Model file for the job. Use its own axes, mm. Round coordinates to 2 decimals unless told otherwise and drop trailing zeros. Order: outer loops, then holes, each group sorted by start corner. A loop starts at its lowest first (then second) coordinate and runs counter-clockwise, first axis right, second up. Notation, with made-up numbers: (-24.75, 15.5) - (2.25, 15.5) arc R29 ccw to (2.25, 37.5) - close; hole circle Ø9 at (0, -0.75). An arc over 180 degrees is marked (long way). Use one line per item in the form item = value.
from build123d import *

# Parameters (mm, degrees)
BOSS_EXTRUDE1_DEPTH  = 22
FILLET1_R            = 5
M4_CLEARANCE_HOLE1_D = 4.3
SKETCH5_R            = 11
CUT_EXTRUDE1_DEPTH   = 22


with BuildPart() as part:
    # Sketch1 → Boss-Extrude1 (new body)
    with BuildSketch(Plane.XY):
        Polygon((0, -21.647844006), (15.307337295, -15.307337295), (21.647844006, 0), (15.307337295, 15.307337295), (0, 21.647844006), (-15.307337295, 15.307337295), (-21.647844006, 0), (-15.307337295, -15.307337295), align=None)
    extrude(amount=BOSS_EXTRUDE1_DEPTH)

    # Fillet1
    fillet1_edges = [part.edges().sort_by_distance(p)[0] for p in [
        (15.307337295, -15.307337295, 11),
        (0, -21.647844006, 11),
        (-15.307337295, -15.307337295, 11),
        (-21.647844006, 0, 11),
        (-15.307337295, 15.307337295, 11),
        (0, 21.647844006, 11),
        (15.307337295, 15.307337295, 11),
        (21.647844006, 0, 11),
    ]]
    fillet(fillet1_edges, radius=FILLET1_R)

    # M4 Clearance Hole1 (through all)
    with Locations(Plane.XY.offset(22)):
        with Locations((0, 16), (16, 0), (0, -16), (-16, 0)):
            Hole(M4_CLEARANCE_HOLE1_D / 2)

    # Sketch5 → Cut-Extrude1 (cut)
    with BuildSketch(Plane.XY.offset(22)):
        Circle(SKETCH5_R)
    extrude(amount=-CUT_EXTRUDE1_DEPTH, mode=Mode.SUBTRACT)


solid = part.part
(1) Pull direction Y, two halves, no side cores. Call faces 1 (the face through (9, -9, 0)), 2 (the face through (13.95, 0.65, 10.85)), 3 (the face through (-2.38, -10.74, 11.15)), 4 (the face through (-7.734, -18.444, 10.846)): released by +Y, released by -Y, zero draft, split by the parting line, or undercut.
Report:
face_1 = zero draft
face_2 = undercut
face_3 = undercut
face_4 = released by -Y
(2) Slice it at B-B on x = 0. Give the cut face in (y, z).
Report:
outline = (-21.24, 0) - (-18.15, 0) - (-18.15, 22) - (-21.24, 22) - close; (-13.85, 0) - (-11, 0) - (-11, 22) - (-13.85, 22) - close; (11, 0) - (13.85, 0) - (13.85, 22) - (11, 22) - close; (18.15, 0) - (21.24, 0) - (21.24, 22) - (18.15, 22) - close
(3) Slice it at A-A on z = 3.75. Give the cut face in (x, y), then the cut area to 3 significant figures.
Report:
outline = (-20.86, -1.91) - (-16.1, -13.39) arc R5 ccw to (-13.39, -16.1) - (-1.91, -20.86) arc R5 ccw to (1.91, -20.86) - (13.39, -16.1) arc R5 ccw to (16.1, -13.39) - (20.86, -1.91) arc R5 ccw to (20.86, 1.91) - (16.1, 13.39) arc R5 ccw to (13.39, 16.1) - (1.91, 20.86) arc R5 ccw to (-1.91, 20.86) - (-13.39, 16.1) arc R5 ccw to (-16.1, 13.39) - (-20.86, 1.91) arc R5 ccw to start; hole circle Ø4.3 at (-16, 0); hole circle Ø22 at (0, 0); hole circle Ø4.3 at (0, -16); hole circle Ø4.3 at (0, 16); hole circle Ø4.3 at (16, 0)
area = 883 mm2
(4) Slice it at D-D on x = -8. Give the cut face in (y, z), then the cut area to 3 significant figures.
Report:
outline = (-18.33, 0) - (-7.55, 0) - (-7.55, 22) - (-18.33, 22) - close; (7.55, 0) - (18.33, 0) - (18.33, 22) - (7.55, 22) - close
area = 475 mm2
(5) Probe probe 1 along Y at (x, z) = (0, 17); probe 2 along X at (y, z) = (1, 12.25); probe 3 along X at (y, z) = (3, 11). List the from-to ranges inside material, lowest first. Write a range as [from, to].
Report:
probe_1 = [-21.24, -18.15], [-13.85, -11], [11, 13.85], [18.15, 21.24]
probe_2 = [-21.13, -17.9], [-14.1, -10.95], [10.95, 14.1], [17.9, 21.13]
probe_3 = [-20.41, -10.58], [10.58, 20.41]
(6) Pin check, flat tips, straight feed: pin 1 (2 mm diameter, centred on x = -9.5, y = -1, fed in from -Z); pin 2 (2 mm diameter, centred on x = 14, z = 19.5, fed in from +Y); pin 3 (3 mm diameter, centred on x = -13.5, z = 13.5, fed in from +Y); pin 4 (3 mm diameter, centred on y = -10.5, z = 14, fed in from +X). Stop position of each tip, or through.
Report:
pin_1 = through
pin_2 = 16.26
pin_3 = 16.68
pin_4 = 17.92
